from build123d import *

# Parameters (mm, degrees)
EXTRUDE_2_DEPTH     = 30
EXTRUDE_START       = -20
EXTRUDE_1_DEPTH     = 20
CUT_EXTRUDE_1_REACH = 53.624


# Read off the part's stored shape, not the designer's step: 拉伸-薄壁1
with BuildPart() as part:
    # 草图1 → 凸台-拉伸2 (new, symmetric)
    with BuildSketch(Plane.XY):
        Polygon((-26, 5), (26, 5), (26, -5), (10, -5), (12.886751346, 0), (-12.886751346, 0), (-10, -5), (-26, -5), align=None)
    extrude(amount=EXTRUDE_2_DEPTH, both=True)

    # 拉伸-薄壁1 outline → 拉伸-薄壁1 (add)
    with BuildSketch(Plane(origin=(26, 0, 0), x_dir=(0, 0, -1), z_dir=(1, 0, 0)).offset(EXTRUDE_START)):
        with BuildLine():
            Line((15, 5), (15, 23))
            ThreePointArc((15, 23), (0, 38), (-15, 23))
            Line((-15, 23), (-15, 5))
            Line((-15, 5), (15, 5))
        make_face()
        with BuildLine():
            ThreePointArc((-10, 23), (0, 33), (10, 23))
            Line((10, 23), (10, 10))
            Line((10, 10), (-10, 10))
            Line((-10, 10), (-10, 23))
        make_face(mode=Mode.SUBTRACT)
    extrude(amount=EXTRUDE_1_DEPTH)

    # 草图6 → 切除-拉伸1 (cut, up to next)
    with BuildSketch(Plane(origin=(0, 5, 0), x_dir=(1, 0, 0), z_dir=(0, 1, 0)), mode=Mode.PRIVATE) as cut_extrude_1_sk1:
        Polygon((-6, -11.607695155), (-12, -8.143593539), (-18, -11.607695155), (-18, -18.535898385), (-12, -22), (-6, -18.535898385), align=None)
    cut_extrude_1_tool1 = extrude(cut_extrude_1_sk1.sketch, amount=-CUT_EXTRUDE_1_REACH, mode=Mode.PRIVATE) & part.part
    add(cut_extrude_1_tool1.solids().sort_by_distance((-12, 5, 15.071797))[0], mode=Mode.SUBTRACT)


solid = part.part
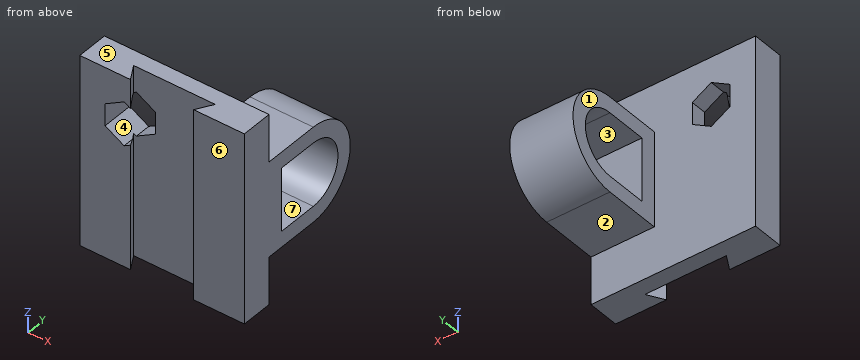
The model under review builds one solid part; all positions refer to its coordinate system, in mm. Face numbers are marked on the shaded views. A direction names the side the tool comes from. Coordinates: 2 decimals unless noted, no trailing zeros. Order: outer loops, then holes, each group sorted by start corner. A loop starts at its lowest first (then second) coordinate and runs counter-clockwise, first axis right, second up. Notation, with made-up numbers: (55, 4) -> (103, 4) arc R29 ccw to (103, 31) -> close; hole circle Ø4 at (45.25, -33.75). An arc over 180 degrees is marked (long way). Answer in a Markdown table with one row per item.
(1) Consider section D-D (z = 0). Write out the cut boundary in (x, y), plus the area to 3 significant figures.
Answers:
| item | result |
|---|---|
| outline | (-26, -5) -> (-10, -5) -> (-12.89, 0) -> (12.89, 0) -> (10, -5) -> (26, -5) -> (26, 10) -> (6, 10) -> (6, 5) -> (-26, 5) -> close; (6, 33) -> (26, 33) -> (26, 38) -> (6, 38) -> close |
| area | 606 mm² |
(2) Consider section C-C (x = 14). Write out the cut boundary in (y, z).
Answers:
| item | result |
|---|---|
| outline | (-5, -30) -> (5, -30) -> (5, -15) -> (23, -15) arc R15 ccw to (23, 15) -> (5, 15) -> (5, 30) -> (-5, 30) -> close; hole (10, -10) -> (23, -10) arc R10 ccw to (23, 10) -> (10, 10) -> close |
(3) Consider section A-A (z = 16). Write out the cut boundary in (x, y), plus the area to 3 significant figures.
Answers:
| item | result |
|---|---|
| outline | (-26, -5) -> (-18, -5) -> (-18, 5) -> (-26, 5) -> close; (-6, 0) -> (12.89, 0) -> (10, -5) -> (26, -5) -> (26, 5) -> (-6, 5) -> close |
| area | 313 mm² |
(4) Machinability: for the marked faces 1, 2, 3 and 4, which of the approach directions +Z, -Z, +X, -X, +Y, -Y give a long, thin tool a straight path to every point of the face, cutting with its end or side? Answer none if there is none.
Answers:
| item | result |
|---|---|
| face 1 | +Z, -Z, -X, +Y |
| face 2 | -Z, +X, -X, +Y |
| face 3 | +X, -X |
| face 4 | +Y, -Y |
(5) Consider section B-B (y = 13.5). Write out the cut boundary in (x, z), plus the area to 3 significant figures.
Answers:
| item | result |
|---|---|
| outline | (6, -15) -> (26, -15) -> (26, -10) -> (6, -10) -> close; (6, 10) -> (26, 10) -> (26, 15) -> (6, 15) -> close |
| area | 200 mm² |
(6) Wall thickness on line 1 along Z through (x, y) = (24, 17); line 2 along Y through (x, z) = (-12, -10.5); line 3 along Y through (x, z) = (0.5, -18): over which ranges is each line inside the solid? List them lowest first.
Answers:
| item | result |
|---|---|
| line 1 | -15 to -10, 10 to 15 |
| line 2 | -5 to -1.54, 0 to 5 |
| line 3 | 0 to 5 |
(7) The part is to be moulded in two halves that separate along Z. For the marked faces 5, 6 and 7, say which applies: +Z half, -Z half, draft (parallel to the pull), parting line (faces both ways), or undercut.
Answers:
| item | result |
|---|---|
| face 5 | +Z half |
| face 6 | draft |
| face 7 | undercut |
(8) Insertion check: pin 1 (8 mm diameter, centred on y = 26.5, z = -8.5, fed in from -X); pin 2 (14.5 mm diameter, centred on x = 21, y = 16.5, fed in from -Z); pin 3 (12 mm diameter, centred on x = 19.5, z = 17.5, fed in from +Y). Each pin has a flat end and moves straight along its axis. Give the tip position at first contact, or say it passes through.
Answers:
| item | result |
|---|---|
| pin 1 | x = 6 |
| pin 2 | z = -15 |
| pin 3 | y = 32.63 |
